Job drawing, mm, ordinate dimensions from the low corner. One solid piece. A direction names the side the tool comes from. Round coordinates to 2 decimals unless told otherwise and drop trailing zeros. Order: outer loops, then holes, each group sorted by start corner. A loop starts at its lowest first (then second) coordinate and runs counter-clockwise, first axis right, second up. Notation, with made-up numbers: (47, 5.25) -> (76, 5.25) arc R15 cw to (76, 26.25) -> close; hole circle Ø10 at (5, 85.25). An arc over 180 degrees is marked (long way). Answer as a JSON object with one key per item and string values. Group by question number.
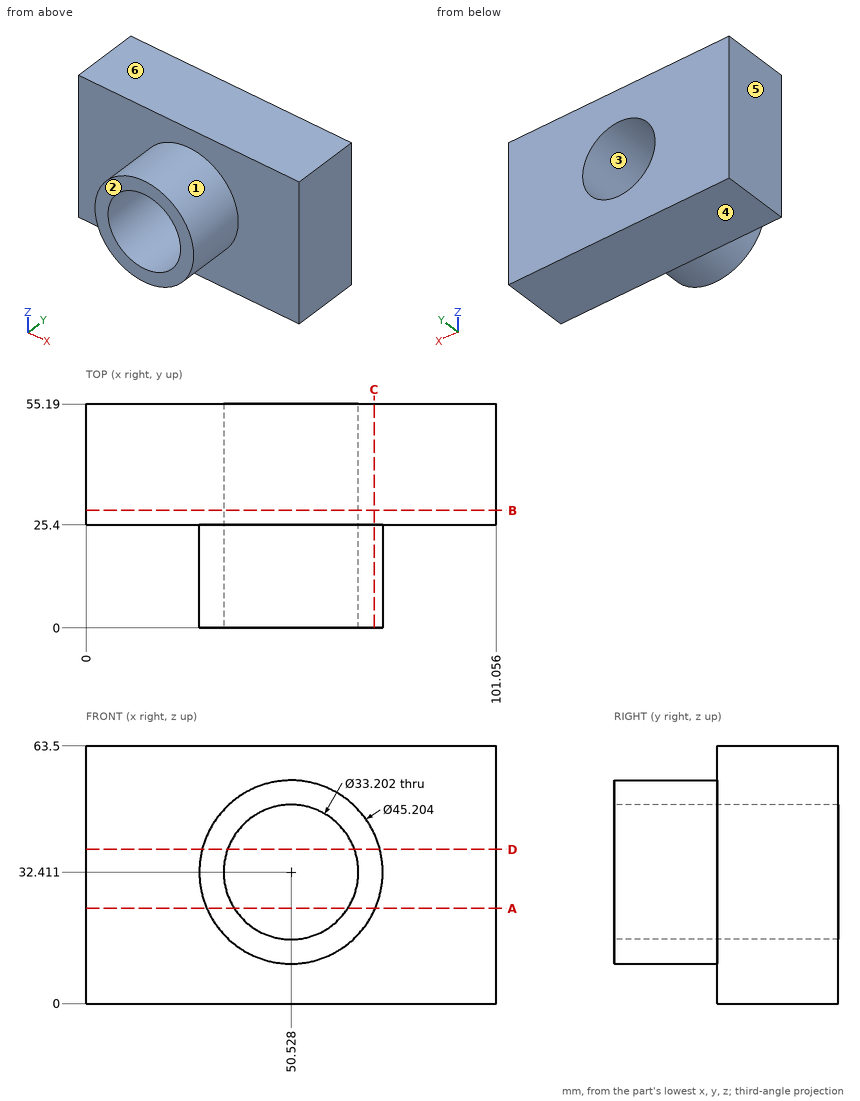
Q1. Band-saw the part on C-C (x = 71). List the corners of the cut face in (y, z), plus the area to 3 significant figures.
Q2. Which spindle directions (+Z, -Z, +X, -X, +Y, -Y) get a long thin tool onto all of the face, cutting with end or side? Do the marked faces 1 and 2. Say none if no direction does.
Q3. Wall check: line 1 (Z direction, x = 49.5, y = 5); line 2 (X direction, y = 43.5, z = 31.5) (1 decimal); line 3 (X direction, y = 6.5, z = 25) (1 decimal). Give the ranges that are in metal, low to high. Write a range as [from, to].
Q4. Band-saw the part on A-A (z = 23.5). List the corners of the cut face in (x, y) (1 decimal), plus the area to 3 significant figures.
Q5. Two-plate mould, pull along Z, no slides. Class the marked faces 3, 4, 5 and 6: +Z half, -Z half, draft (parallel to the pull), parting line (faces both ways), or undercut.
Q6. Band-saw the part on B-B (y = 29). List the corners of the cut face in (x, z) (1 decimal).
Q7. Drop flat-ended pins along their axis: pin 1 Ø20 at (x, z) = (50.53, 32.41) entering from +Y; pin 2 Ø6 at (x, z) = (14, 35.5) entering from -Y. Give the stop position or say it passes through.
Q8. Band-saw the part on D-D (z = 38). List the corners of the cut face in (x, y) (1 decimal).
Completed:
{
 "1": {"outline": "(0, 22.83) -> (25.4, 22.83) -> (25.4, 0) -> (55.19, 0) -> (55.19, 63.5) -> (25.4, 63.5) -> (25.4, 41.99) -> (0, 41.99) -> close", "area": "2,380 mm2"},
 "2": {"face 1": "-Y", "face 2": "+Z, -Z, +X, -X, -Y"},
 "3": {"line 1": "[9.83, 15.84], [48.98, 54.99]", "line 2": "[0, 34], [67.1, 101.1]", "line 3": "[29.2, 35.7], [65.4, 71.9]"},
 "4": {"outline": "(0, 25.4) -> (29.8, 25.4) -> (29.8, 0) -> (36.5, 0) -> (36.5, 55.2) -> (0, 55.2) -> close; (64.5, 0) -> (71.3, 0) -> (71.3, 25.4) -> (101.1, 25.4) -> (101.1, 55.2) -> (64.5, 55.2) -> close", "area": "2,520 mm2"},
 "5": {"face 3": "undercut", "face 4": "-Z half", "face 5": "draft", "face 6": "+Z half"},
 "6": {"outline": "(0, 0) -> (101.1, 0) -> (101.1, 63.5) -> (0, 63.5) -> close; hole circle Ø33.2 at (50.5, 32.4)"},
 "7": {"pin 1": "through", "pin 2": "y = 25.4"},
 "8": {"outline": "(0, 25.4) -> (28.6, 25.4) -> (28.6, 0) -> (34.9, 0) -> (34.9, 55.2) -> (0, 55.2) -> close; (66.2, 0) -> (72.4, 0) -> (72.4, 25.4) -> (101.1, 25.4) -> (101.1, 55.2) -> (66.2, 55.2) -> close"}
}
